```python
from build123d import *

# Parameters (mm, degrees)
PAD_DEPTH        = 3
CHAMFER_SIZE2    = 1
CHAMFER_SIZE     = 5.5
CHAMFER001_SIZE2 = 5.5
CHAMFER001_SIZE  = 1


with BuildPart() as part:
    # Sketch → Pad (new body)
    with BuildSketch(Plane.XY):
        with BuildLine():
            Line((-9.971835, 0.75), (-4, 0.75))
            Line((-4, 0.75), (-4, 1.5))
            Line((-4, 1.5), (4, 1.5))
            Line((4, 1.5), (4, -1.5))
            Line((4, -1.5), (-4, -1.5))
            Line((-4, -1.5), (-4, -0.75))
            Line((-4, -0.75), (-9.971835, -0.75))
            ThreePointArc((-9.971835, -0.75), (10, 0), (-9.971835, 0.75))
        make_face()
    extrude(amount=PAD_DEPTH)

    # Chamfer
    chamfer_edges = [part.edges().sort_by_distance(p)[0] for p in [
        (-9.971835, 0.75, 1.5),
    ]]
    chamfer_side = part.faces().sort_by_distance((-6.985918, 0.75, 1.5))[0]
    chamfer(chamfer_edges, length=CHAMFER_SIZE, length2=CHAMFER_SIZE2, reference=chamfer_side)

    # Chamfer001
    chamfer001_edges = [part.edges().sort_by_distance(p)[0] for p in [
        (-9.971835, -0.75, 1.5),
    ]]
    chamfer001_side = part.faces().sort_by_distance((9.987492, -0.5, 1.5))[0]
    chamfer(chamfer001_edges, length=CHAMFER001_SIZE, length2=CHAMFER001_SIZE2, reference=chamfer001_side)


solid = part.part
```
Source: CAD feature listing. Evaluate the final solid. Frame: model axes, mm. A direction names the side the tool comes from. Coordinates: 2 decimals unless noted, no trailing zeros. Loops run counter-clockwise (first coordinate to the right, second up) from the corner with the lowest first, then second, coordinate; pieces in that order, holes last. Notation, with made-up numbers: M 64,88 L 75,88 A15 cw 75,115 Z; hole C -14,62.5 d10. An arc over 180 degrees is marked long. Use a Markdown table: item, result. Add a question column.
Q1. Access query for faces 4 (the flat face through (-7.12, -1.24, 1.48)), 5 (the flat face through (0, -2, 3)), 6 (the flat face through (4, 0, 1)). Directions: +Z, -Z, +X, -X, +Y, -Y. A direction counts if a zero-diameter tool reaches every point of the face in a straight line with its end or side. Return the directions, or none.
Q2. Section query C-C, the plane x = -8.25. Return loops of the section in (y, z).
Q3. First-contact query: pin 1 (0.6 mm diameter, centred on y = -1.5, z = 2, fed in from +X); pin 2 (1 mm diameter, centred on x = -6.5, z = 1.5, fed in from -Y); pin 3 (0.5 mm diameter, centred on x = -4, z = 1.5, fed in from -Y). Flat tips, straight axial feed; report the tip coordinate or a pass-through.
Q4. Section query D-D, the plane y = 0. Return loops of the section in (x, z).
Q5. Section query B-B, the plane z = 2.6. Return loops of the section in (x, y), and give its area (3 significant figures).
Q6. Draft query along X for faces 1 (the flat face through (0, 1.5, 1)), 2 (the flat face through (-7.197, 1.253, 1.479)), 3 (the flat face through (0, -2, 0)). Return one class per face: pulls with the +X half, pulls with the -X half, needs draft (parallel to the pull), parting line crosses it, or undercut.
Q7. Material intervals for L1, parallel to Y at x = 2, z = 0.7; L2, parallel to Y at x = -7.25, z = 1.1; L3, parallel to X at y = 0, z = 1.45, sorted ascending.
Q8. Section query A-A, the plane x = 0. Return loops of the section in (y, z), and give its area (3 significant figures).
Result:
| question | item | result |
|---|---|---|
| 1 | face 4 | +Z, -Z, -X |
| 1 | face 5 | +Z, +X, -X, +Y, -Y |
| 1 | face 6 | +Z, -Z |
| 2 | outline | M -5.65,0 L -1.45,0 L -1.45,3 L -5.65,3 Z; M 1.45,0 L 5.65,0 L 5.65,3 L 1.45,3 Z |
| 3 | pin 1 | stops at x = 9.93 |
| 3 | pin 2 | stops at y = -8 |
| 3 | pin 3 | stops at y = -9.27 |
| 4 | outline | M 4,0 L 10,0 L 10,3 L 4,3 Z |
| 5 | outline | M -9.85,-1.74 A10 ccw long -9.85,1.74 L -4.47,0.75 L -4,0.75 L -4,1.5 L 4,1.5 L 4,-1.5 L -4,-1.5 L -4,-0.75 L -4.47,-0.75 Z |
| 5 | area | 276 mm2 |
| 6 | face 1 | undercut |
| 6 | face 2 | pulls with the -X half |
| 6 | face 3 | needs draft |
| 7 | L1 | y = -9.8 to -1.5, 1.5 to 9.8 |
| 7 | L2 | y = -6.89 to -1.26, 1.26 to 6.89 |
| 7 | L3 | x = 4 to 10 |
| 8 | outline | M -10,0 L -1.5,0 L -1.5,3 L -10,3 Z; M 1.5,0 L 10,0 L 10,3 L 1.5,3 Z |
| 8 | area | 51.0 mm2 |
